Part model, mm, in its own coordinate system. Coordinates: 2 decimals unless noted, no trailing zeros. Loops run counter-clockwise (first coordinate to the right, second up) from the corner with the lowest first, then second, coordinate; pieces in that order, holes last. Notation, with made-up numbers: (-34.75, 24.25) -> (-6.75, 24.25) arc R19 cw to (-6.75, 38.25) -> close; hole circle Ø10 at (-34.5, 20). An arc over 180 degrees is marked (long way). Use one line per item in the form item = value. Start each with the question number.
(1) Band-saw the part on C-C on x = -8.75. Count the separate pieces of the cut face and the enclosed holes in it, then the cut area to 3 significant figures.
(2) Drill centre lines: L1, parallel to Y at x = -2.5, z = 43.5; L2, parallel to Z at x = -6.5, y = 4.5; L3, parallel to Z at x = -10.5, y = 40. Where is each one in solid material? Low to high. Write a range as [from, to].
(3) Band-saw the part on B-B on z = -24. Give the cut face in (x, y), then the cut area to 3 significant figures.
(4) Band-saw the part on A-A on y = 0. Give the cut face in (x, z).
```python
from build123d import *

# Parameters (mm, degrees)
F0_W     = 120
F0_H     = 240
F0_R     = 1.75
F0_R_2   = 51.75
F0_R_3   = 1.25
F1_DEPTH = 15


# Not quite as in the source:
# - a feature names something its author has since deleted; it is built from what else it names


with BuildPart() as f1:
    # F0 (on Right) → F1 (new body)
    with BuildSketch(Plane.YZ):
        with Locations((0, 4.9354011911)):
            Rectangle(F0_W, F0_H)
        with Locations((-49.9999973178, -107.0645988089)):
            Circle(F0_R, mode=Mode.SUBTRACT)
        with Locations((-40.3050865276, -83.1196853366)):
            Circle(F0_R, mode=Mode.SUBTRACT)
        with Locations((-40.3050865276, -2.5095122813)):
            Circle(F0_R, mode=Mode.SUBTRACT)
        with Locations((50.0000026822, -107.0645988089)):
            Circle(F0_R, mode=Mode.SUBTRACT)
        with Locations((40.3050865276, -83.1196853366)):
            Circle(F0_R, mode=Mode.SUBTRACT)
        with Locations((0, -42.8145988089)):
            Circle(F0_R_2, mode=Mode.SUBTRACT)
        with Locations((40.3050865276, -2.5095122813)):
            Circle(F0_R, mode=Mode.SUBTRACT)
        with Locations((-28.8463527312, 31.4634012507)):
            Circle(F0_R_3, mode=Mode.SUBTRACT)
        with Locations((-45.6305965781, 65.8711940348)):
            Circle(F0_R_3, mode=Mode.SUBTRACT)
        with Locations((-49.9999973178, 116.9354011911)):
            Circle(F0_R, mode=Mode.SUBTRACT)
        with BuildLine():
            ThreePointArc((-22.0790897047, 101.9354011911), (-21.2004100483, 104.0567215346), (-19.0790897047, 104.9354011911))
            Line((-19.0790897047, 104.9354011911), (18.9209102953, 104.9354011911))
            ThreePointArc((18.9209102953, 104.9354011911), (21.0422306388, 104.0567215346), (21.9209102953, 101.9354011911))
            Line((21.9209102953, 101.9354011911), (21.9209102953, 29.9354011911))
            ThreePointArc((21.9209102953, 29.9354011911), (21.0422306388, 27.8140808475), (18.9209102953, 26.9354011911))
            Line((18.9209102953, 26.9354011911), (-19.0790897047, 26.9354011911))
            ThreePointArc((-19.0790897047, 26.9354011911), (-21.2004100483, 27.8140808475), (-22.0790897047, 29.9354011911))
            Line((-22.0790897047, 29.9354011911), (-22.0790897047, 101.9354011911))
        make_face(mode=Mode.SUBTRACT)
        with Locations((-28.8463527312, 100.4074011314)):
            Circle(F0_R_3, mode=Mode.SUBTRACT)
        with Locations((28.8463527312, 31.4634012507)):
            Circle(F0_R_3, mode=Mode.SUBTRACT)
        with Locations((28.8463527312, 100.4074011314)):
            Circle(F0_R_3, mode=Mode.SUBTRACT)
        with Locations((45.0773127377, 65.8711940348)):
            Circle(F0_R_3, mode=Mode.SUBTRACT)
        with Locations((50.0000026822, 116.9354046481)):
            Circle(F0_R, mode=Mode.SUBTRACT)
    extrude(amount=-F1_DEPTH)


solid = f1.part
```
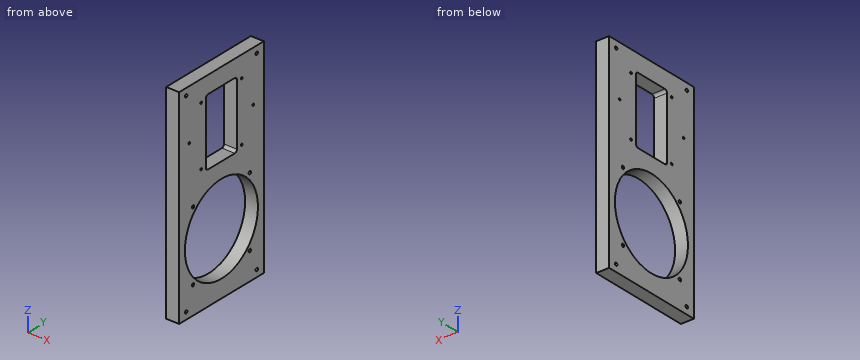
A:
q1.separate_pieces = 1
q1.enclosed_holes = 16
q1.area = 16,900 mm²
q2.L1 = [-60, -22.08], [21.92, 60]
q2.L2 = [-115.06, -94.37], [8.74, 26.94], [104.94, 124.94]
q2.L3 = [-115.06, -84.84], [-81.4, -75.65], [-9.98, -4.23], [-0.79, 124.94]
q3.outline = (-15, -60) -> (0, -60) -> (0, -48.21) -> (-15, -48.21) -> close; (-15, 48.21) -> (0, 48.21) -> (0, 60) -> (-15, 60) -> close
q3.area = 354 mm²
q4.outline = (-15, -115.06) -> (0, -115.06) -> (0, -94.56) -> (-15, -94.56) -> close; (-15, 8.94) -> (0, 8.94) -> (0, 26.94) -> (-15, 26.94) -> close; (-15, 104.94) -> (0, 104.94) -> (0, 124.94) -> (-15, 124.94) -> close
